```python
from build123d import *

# Parameters (mm, degrees)
BOSS_EXTRUDE1_DEPTH = 431.8
SKETCH4_W           = 15.875
SKETCH4_H           = 25.4
CUT_EXTRUDE1_DEPTH  = 6.35
SKETCH5_W           = 1.5875
SKETCH5_H           = 25.4
CUT_EXTRUDE2_DEPTH  = 6.35


with BuildPart() as part:
    # Sketch2 → Boss-Extrude1 (new body)
    with BuildSketch(Plane(origin=(0, 0, 0), x_dir=(1, 0, 0), z_dir=(0, 1, 0))):
        with BuildLine():
            Line((0, 0), (19.05, 0))
            Line((19.05, 0), (19.05, 1.5875))
            ThreePointArc((19.05, 1.5875), (18.585032015, 2.710032015), (17.4625, 3.175))
            Line((17.4625, 3.175), (4.7625, 3.175))
            ThreePointArc((4.7625, 3.175), (3.639967985, 3.639967985), (3.175, 4.7625))
            Line((3.175, 4.7625), (3.175, 17.4625))
            ThreePointArc((3.175, 17.4625), (2.710032015, 18.585032015), (1.5875, 19.05))
            Line((1.5875, 19.05), (0, 19.05))
            Line((0, 19.05), (0, 0))
        make_face()
    extrude(amount=BOSS_EXTRUDE1_DEPTH)

    # Sketch4 → Cut-Extrude1 (cut)
    with BuildSketch(Plane(origin=(3.175, 0, 0), x_dir=(0, 0, -1), z_dir=(1, 0, 0))):
        with Locations((11.1125, 419.1)):
            Rectangle(SKETCH4_W, SKETCH4_H)
    extrude(amount=-CUT_EXTRUDE1_DEPTH, mode=Mode.SUBTRACT)

    # Sketch5 → Cut-Extrude2 (cut)
    with BuildSketch(Plane.ZY.offset(-3.175)):
        with Locations((-3.96875, 419.1)):
            Rectangle(SKETCH5_W, SKETCH5_H)
    extrude(amount=-CUT_EXTRUDE2_DEPTH, mode=Mode.SUBTRACT)


solid = part.part
```
The listing builds one solid part. Answer for the finished solid, in the listing's coordinates (mm). A direction names the side the tool comes from. Coordinates: 2 decimals unless noted, no trailing zeros. Loops run counter-clockwise (first coordinate to the right, second up) from the corner with the lowest first, then second, coordinate; pieces in that order, holes last. Notation, with made-up numbers: (-38.5, 53.25) - (16.5, 53.25) arc R21 ccw to (16.5, 60.25) - close; hole circle Ø1 at (65, 16.25). An arc over 180 degrees is marked (long way). Write item = value, one per line.
1) Find the intervals of material crossed by line 1 along Z through (x, y) = (16, 221.5) (3 decimals); line 2 along X through (y, z) = (27, -15.5) (3 decimals); line 3 along Y through (x, z) = (1.25, -13.5), in increasing order.
Responses:
line_1 = -3.175 to 0
line_2 = 0 to 3.175
line_3 = 0 to 406.4
2) Which of the six approach directions +Z, -Z, +X, -X, +Y, -Y give full straight-line access (tool end or side, diameter ignored) to faces 1 (the face through (3, 0, -6)), 2 (the face through (3.175, 200, -11))?
Responses:
face_1 = +Z, -Z, +X, -X, -Y
face_2 = -Z, +X, +Y, -Y
3) Section B-B (z = -14.25) is taken. Determine the outline of the cut face in (x, y) (3 decimals).
Responses:
outline = (0, 0) - (3.175, 0) - (3.175, 406.4) - (0, 406.4) - close
4) Each of these flat-tipped pins is pushed along its axis until it touches: P1, Ø8, axis at x = 11.5, y = 260, coming from the +Z side; P2, Ø6, axis at x = 2, z = -13, coming from the +Y side; P3, Ø1, axis at x = 12.5, y = 45.5, coming from the -Z side (3 decimals). Where does it stop, or does it pass through?
Responses:
P1 = 0
P2 = 406.4
P3 = -3.175
